Input: part model. Units: mm. Frame: model coordinates. Give positions to 0.01 mm unless a question says otherwise; leave off trailing zeros. Write each loop counter-clockwise with the first axis right and the second up, starting at its lowest first coordinate (ties: lowest second). Pieces come first, ordered by that corner, then holes.
```python
from build123d import *

# Parameters (mm, degrees)
F1_DEPTH = 100.2740859985
F3_D     = 7.5
F3_DEPTH = 2
F3_TIP   = 2.2532273214


with BuildPart() as f1:
    # F0 (on Front) → F1 (new body)
    with BuildSketch(Plane.XZ):
        Polygon((-8.5613747377, 8.1151898103), (-46.5092712761, 44.0853923477), (-27.2959015118, -9.0020827425), align=None)
        Polygon((-47.045001057, 45.5656397871), (-46.5092712761, 44.0853923477), (-8.5613747377, 8.1151898103), (27.9545485973, 41.4788834751), (-12.6136355102, 78.3473849297), align=None)
    extrude(amount=F1_DEPTH)

    # F3
    with Locations(Plane(origin=(-45.1239530897, 0, 47.3946495829), x_dir=(0.7242433012, 0, 0.6895445168), z_dir=(-0.6895445168, 0, 0.7242433012))):
        with Locations((21.8701027334, -45.7103922963)):
            Hole(F3_D / 2, depth=F3_DEPTH)
            with Locations((0, 0, -(F3_DEPTH + F3_TIP / 2))):  # 118° drill point
                Cone(0, F3_D / 2, F3_TIP, mode=Mode.SUBTRACT)


solid = f1.part
```
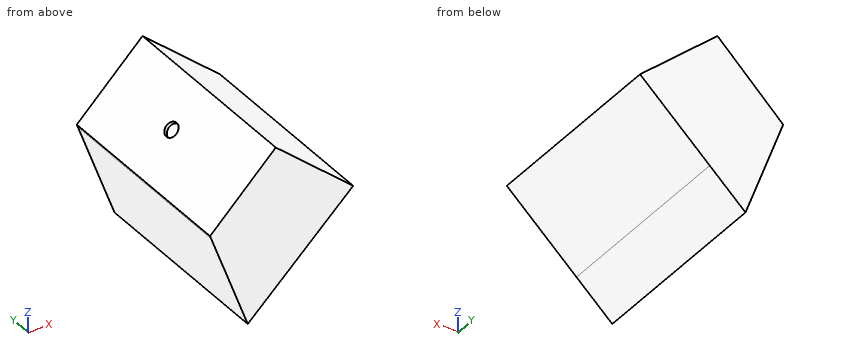
Q1. Section A-A, the plane y = -83. Return the cut outline in (x, z) (3 decimals), then the cut area to 3 significant figures.
Q2. Material intervals for line 1 along Z through (x, y) = (22, -60); line 2 along X through (y, z) = (-9, 58); line 3 along X through (y, z) = (-42, 1.5), sorted ascending.
Q3. Section C-C, the plane z = 38. Return the cut outline in (x, y).
Q4. Section B-B, the plane x = -34. Return the cut outline in (y, z), then the cut area to 3 significant figures.
Q5. Pin query (flat end, axial travel): pin 1 (10 mm diameter, centred on x = 19, y = -78, fed in from -Z); pin 2 (12 mm diameter, centred on x = -13, y = -20.5, fed in from -Z); pin 3 (6 mm diameter, centred on y = -17, z = 0.5, fed in from +X). Return the tip coordinate at first contact, or that it passes through.
Solutions:
1. outline: (-47.045, 45.566) - (-27.296, -9.002) - (27.955, 41.479) - (-12.614, 78.347) - close
1. area: 3,310 mm2
2. line 1: z = 36.04 to 46.89
2. line 2: x = -33.98 to 9.78
2. line 3: x = -31.1 to -15.8
3. outline: (-44.31, -100.27) - (24.15, -100.27) - (24.15, 0) - (-44.31, 0) - close
4. outline: (-100.27, 9.52) - (0, 9.52) - (0, 57.99) - (-100.27, 57.99) - close
4. area: 4,860 mm2
5. pin 1: stops at z = 28.73
5. pin 2: stops at z = -1.42
5. pin 3: stops at x = -13.61
